Autodesk Fusion 360 part; units mm, degrees
sketch "Sketch1" plane through (0, 0, 0) normal (0, 0, 1) x (1, 0, 0)
  line L0 (44, 40) -> (-44, 40)
  line L1 (-44, 40) -> (-44, -40)
  line L2 (44, -40) -> (44, 40)
  circle A0 centre (25, -4) radius 5
  circle A1 centre (-25, -4) radius 5
  arc A2 (-13.8302, -53.0279) -> (13.8302, -53.0279) centre (0, -40) ccw
  line L3 (-44, -40) -> (-13.8302, -53.0279)
  line L4 (13.8302, -53.0279) -> (44, -40)
  dimension "d1" = 88
  dimension "d2" = 80
  dimension "d7" = 10
  dimension "d8" = 10
  dimension "d9" = 19
extrude "Extrude1" add sketch "Sketch1" along normal blind 10
chamfer "Chamfer1" distance 32.8 angle 45 2 edges at (-44, -40, 5) (44, -40, 5)
fillet "Fillet1" radius 13 2 edges at (-44, -7.2, 5) (44, -7.2, 5)
sketch "Sketch2" plane through (0, 0, 0) normal (1, 0, 0) x (0, 1, 0)
  line L0 (40, 10) -> (40, 0) construction
  line L1 (20, 10) -> (20, 50)
  line L2 (20, 10) -> (-44, 10)
  line L3 (20, 50) -> (-44, 10)
  dimension "d15" = 20
  dimension "d16" = 64
  dimension "d17" = 40
extrude "Extrude2" add sketch "Sketch2" along normal mid plane 10
sketch "Sketch3" plane through (0, 0, 0) normal (0, 0, 1) x (1, 0, 0)
  line L0 (-44, 40.1) -> (-44, 27.1)
  line L1 (44, 27.1) -> (44, 40.1)
  circle A0 centre (0, 46.1) radius 9.5
  line L2 (5, 23.7404) -> (16, 23.7404)
  line L3 (16, 23.7404) -> (5, 23.7404)
  line L4 (-5, 23.7404) -> (-16, 23.7404)
  line L5 (-16, 23.7404) -> (-16, 27.1)
  line L6 (16, 23.7404) -> (16, 27.1)
  line L7 (5, 20) -> (5, 23.7404)
  line L8 (-5, 20) -> (-5, 23.7404)
  arc A1 (18.0278, 40.1) -> (-18.0278, 40.1) centre (0, 46.1) ccw
  line L9 (-5, 20) -> (5, 20)
  line L10 (44, 40.1) -> (18.0278, 40.1)
  line L11 (-18.0278, 40.1) -> (-44, 40.1)
  line L12 (-44, 27.1) -> (-16, 27.1)
  line L13 (16, 27.1) -> (44, 27.1)
  dimension "d20" = 13
  dimension "d22" = 19
  dimension "d23" = 19
extrude "Extrude3" add sketch "Sketch3" along normal blind 50
fillet "Fillet2" radius 3 2 edges at (-16, 23.7404, 30) (16, 23.7404, 30)
equation "d2 = 67 mm + 13 mm"
Read the model definition and answer for the solid it produces. Units are mm, in the model's axes. A direction names the side the tool comes from. Round coordinates to 2 decimals unless told otherwise and drop trailing zeros. Write each loop counter-clockwise with the first axis right and the second up, starting at its lowest first coordinate (ties: lowest second). Pieces come first, ordered by that corner, then holes.
1. Given pin 1 Ø4 at (x, z) = (-8.5, 20) entering from -Y; pin 2 Ø8.5 at (x, z) = (24.5, 26) entering from -Y; pin 3 Ø6 at (x, z) = (-22, 6) entering from -Y, each flat-ended and moving along its own axis, determine where each tip first touches the part or whether it passes through.
2. The part is cut by section D-D, the plane z = 24. Determine the outline of the cut face in (x, y).
3. The part is cut by section A-A, the plane x = 0. Determine the outline of the cut face in (y, z), then the cut area to 3 significant figures.
4. Determine the mould class of faces 1 (the face through (0, -12, 30)), 2 (the face through (-0.503, 65.093, 24.65)), 3 (the face through (44, 28, 19)) for opening direction Y: pulls with the +Y half, pulls with the -Y half, needs draft (parallel to the pull), parting line crosses it, or undercut.
5. The part is cut by section C-C, the plane y = 46.1. Determine the outline of the cut face in (x, z).
6. The part is cut by section B-B, the plane z = 16.5. Determine the outline of the cut face in (x, y).
7. Which of the six approach directions +Z, -Z, +X, -X, +Y, -Y give full straight-line access (tool end or side, diameter ignored) to faces 4 (the face through (-5, -3, 25)), 5 (the face through (9, 23.74, 30)), 6 (the face through (4.38, 54.53, 24.65))?
8. Straight lines are drawn through the part: L1, parallel to X at y = 46.1, z = 14; L2, parallel to Z at x = -35, y = 26; L3, parallel to X at y = 18.5, z = 29.5. For each, find the intervals that lie inside material, in ascending order.
Values:
1. pin 1: stops at y = 23.74
1. pin 2: stops at y = 27.1
1. pin 3: stops at y = -45.23
2. outline: (-44, 27.1) - (-16, 27.1) - (-16, 26.74) arc R3 ccw to (-13, 23.74) - (-5, 23.74) - (-5, -21.6) - (5, -21.6) - (5, 23.74) - (13, 23.74) arc R3 ccw to (16, 26.74) - (16, 27.1) - (44, 27.1) - (44, 40.1) - (18.03, 40.1) arc R19 ccw (long way) to (-18.03, 40.1) - (-44, 40.1) - close; hole circle Ø19 at (0, 46.1)
3. outline: (-59, 0) - (40, 0) - (40, 10) - (36.6, 10) - (36.6, 50) - (20, 50) - (-44, 10) - (-59, 10) - close; (55.6, 0) - (65.1, 0) - (65.1, 50) - (55.6, 50) - close
3. area: 3,410 mm2
4. face 1: pulls with the -Y half
4. face 2: undercut
4. face 3: needs draft
5. outline: (-19, 0) - (-9.5, 0) - (-9.5, 50) - (-19, 50) - close; (9.5, 0) - (19, 0) - (19, 50) - (9.5, 50) - close
6. outline: (-44, 27.1) - (-16, 27.1) - (-16, 26.74) arc R3 ccw to (-13, 23.74) - (-5, 23.74) - (-5, -33.6) - (5, -33.6) - (5, 23.74) - (13, 23.74) arc R3 ccw to (16, 26.74) - (16, 27.1) - (44, 27.1) - (44, 40.1) - (18.03, 40.1) arc R19 ccw (long way) to (-18.03, 40.1) - (-44, 40.1) - close; hole circle Ø19 at (0, 46.1)
7. face 4: +Z, -X, -Y
7. face 5: +Z, +X, -Y
7. face 6: +Z
8. L1: x = -19 to -9.5, 9.5 to 19
8. L2: z = 0 to 10
8. L3: x = -5 to 5
